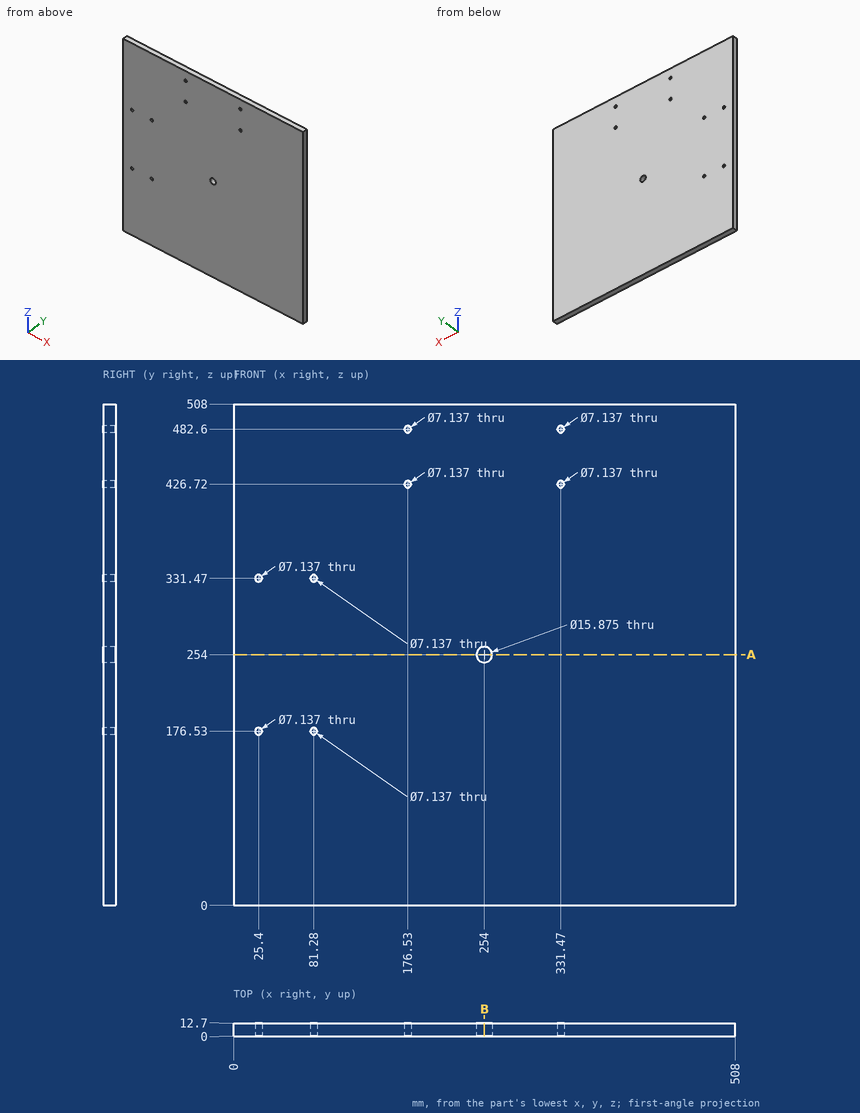
The figure shows three views and two pictorial views of one solid part (mm, origin at its lowest corner). Answer the questions. Coordinates: 2 decimals unless noted, no trailing zeros. Loops run counter-clockwise (first coordinate to the right, second up) from the corner with the lowest first, then second, coordinate; pieces in that order, holes last. Notation, with made-up numbers: (75, -3) - (134, -3) arc R20 ccw to (134, 19) - close; hole circle Ø11 at (89.25, 88). An arc over 180 degrees is marked (long way). Use a Markdown table: item, result. Add a question column.
1) Find the intervals of material crossed by line 1 (X direction, y = 3.25, z = 426.72); line 2 (Z direction, x = 176.53, y = 7.5), in increasing order.
2) The part is cut by section B-B, the plane x = 254. Give the vertices of the cut face in (y, z).
3) The part is cut by section A-A, the plane z = 254. Give the vertices of the cut face in (x, y), and give its area (3 significant figures).
4) Given pin 1 (1 mm diameter, centred on x = 238.5, z = 439, fed in from -Y); pin 2 (12.5 mm diameter, centred on x = 254, z = 254, fed in from +Y), each flat-ended and moving along its own axis, determine where each tip first touches the part or whether it passes through.
Here are the results:
| question | item | result |
|---|---|---|
| 1 | line 1 | x = 0 to 172.96, 180.1 to 327.9, 335.04 to 508 |
| 1 | line 2 | z = 0 to 423.15, 430.29 to 479.03, 486.17 to 508 |
| 2 | outline | (0, 0) - (12.7, 0) - (12.7, 246.06) - (0, 246.06) - close; (0, 261.94) - (12.7, 261.94) - (12.7, 508) - (0, 508) - close |
| 3 | outline | (0, 0) - (246.06, 0) - (246.06, 12.7) - (0, 12.7) - close; (261.94, 0) - (508, 0) - (508, 12.7) - (261.94, 12.7) - close |
| 3 | area | 6,250 mm^2 |
| 4 | pin 1 | stops at y = 0 |
| 4 | pin 2 | passes through |
